Geometry: final body of the model. Coordinates: model frame, mm. Give positions to 0.01 mm unless a question says otherwise; leave off trailing zeros. Write each loop counter-clockwise with the first axis right and the second up, starting at its lowest first coordinate (ties: lowest second). Pieces come first, ordered by that corner, then holes.
Q1. Cut plane C-C on y = 21. Return the cut outline in (x, z), plus the area to 3 significant figures.
Q2. Line query: L1, parallel to Y at x = 0, z = 1.7; L2, parallel to X at y = 10.5, z = 2.05; L3, parallel to Y at x = 0, z = 2.5. Output: solid intervals per line, ascending.
Q3. Cut plane A-A on y = 7. Return the cut outline in (x, z).
Q4. Draft query along Y for faces 1 (the face through (0, 15, 0)), 2 (the face through (0, 5, 1)), 3 (the face through (-3.57, 28.5, 1.51)). Return one class per face: pulls with the +Y half, pulls with the -Y half, needs draft (parallel to the pull), parting line crosses it, or undercut.
Q5. Pin query (flat end, axial travel): pin 1 (3 mm diameter, centred on x = 0, y = 7, fed in from -Z). Return the tip coordinate at first contact, or that it passes through.
```python
from build123d import *

# Parameters (mm, degrees)
F0_W           = 10
F0_H           = 30
F1_DEPTH       = 3
F2_D           = 3.5
F2_DEPTH       = 3
F2_CSINK_D     = 6
F2_CSINK_ANGLE = 90
F2_TIP         = 1.0515060833
F3_R           = 4.99999
F4_R           = 1


# Not quite as in the source:
# - a fillet or chamfer is up to 0.001 mm smaller than in the source, because OpenCascade refuses the exact size


with BuildPart() as f1:
    # F0 (on Top) → F1 (new body)
    with BuildSketch(Plane.XY):
        with Locations((0, 15)):
            Rectangle(F0_W, F0_H)
    extrude(amount=F1_DEPTH)

    # F2
    with Locations(Plane(origin=(0, 0, 0), x_dir=(1, 0, 0), z_dir=(0, 0, -1))):
        with Locations((0, -7)):
            CounterSinkHole(F2_D / 2, F2_CSINK_D / 2, depth=F2_DEPTH, counter_sink_angle=F2_CSINK_ANGLE)
            with Locations((0, 0, -(F2_DEPTH + F2_TIP / 2))):  # 118° drill point
                Cone(0, F2_D / 2, F2_TIP, mode=Mode.SUBTRACT)

    # F3 (radius 5 in the source; OpenCascade refuses exactly that, so slightly less here)
    f3_edges = [f1.edges().sort_by_distance(p)[0] for p in [
        (5, 30, 1.5),
        (-5, 30, 1.5),
    ]]
    fillet(f3_edges, radius=F3_R)

    # F4
    f4_edges = [f1.edges().sort_by_distance(p)[0] for p in [
        (3.535537, 28.535537, 0),
        (3.535537, 28.535537, 3),
        (-5, 12.500005, 3),
        (5, 12.500005, 3),
    ]]
    fillet(f4_edges, radius=F4_R)


solid = f1.part
```
Data:
1. outline: (-5, 1) arc R1 ccw to (-4, 0) - (4, 0) arc R1 ccw to (5, 1) - (5, 2) arc R1 ccw to (4, 3) - (-4, 3) arc R1 ccw to (-5, 2) - close
1. area: 29.1 mm2
2. L1: y = 0 to 5.25, 8.75 to 30
2. L2: x = -5 to 5
2. L3: y = 0 to 5.25, 8.75 to 29.87
3. outline: (-5, 1) arc R1 ccw to (-4, 0) - (-3, 0) - (-1.75, 1.25) - (-1.75, 3) - (-4, 3) arc R1 ccw to (-5, 2) - close; (1.75, 1.25) - (3, 0) - (4, 0) arc R1 ccw to (5, 1) - (5, 2) arc R1 ccw to (4, 3) - (1.75, 3) - close
4. face 1: needs draft
4. face 2: undercut
4. face 3: pulls with the +Y half
5. pin 1: passes through
